```python
from build123d import *

# Parameters (mm, degrees)
F1_DEPTH = 100
F3_DEPTH = 100
F4_W     = 37.074
F4_H     = 23.256904
F4_H_2   = 25
F5_DEPTH = 150
F7_DEPTH = 25


with BuildPart() as f1:
    # F0 (on Front) → F1 (new body)
    with BuildSketch(Plane.XZ):
        Polygon((0, 90), (0, 0), (148.54021, 0), (148.54021, 110.875965), align=None)
    extrude(amount=F1_DEPTH)

    # F2 (on face) → F3 (cut)
    with BuildSketch(Plane.XZ.offset(100)):
        Polygon((7, 0), (40, 0), (148.54021, 0), (148.54021, 169.224784), (40, 169.224784), (40, 95.621633), (7, 57.987016), align=None)
    extrude(amount=-F3_DEPTH, mode=Mode.SUBTRACT)

    # F4 (on face) → F5 (cut)
    with BuildSketch(Plane(origin=(0, 0, 0), x_dir=(1, 0, 0), z_dir=(0, 0, -1))):
        with Locations((25.537, 8.371548)):
            Rectangle(F4_W, F4_H)
        with Locations((25.537, 42.5)):
            Rectangle(F4_W, F4_H_2)
        with Locations((25.537, 77.5)):
            Rectangle(F4_W, F4_H_2)
    extrude(amount=-F5_DEPTH, mode=Mode.SUBTRACT)

    # F6 (on face) → F7 (cut)
    with BuildSketch(Plane.YZ.offset(7)):
        with BuildLine():
            ThreePointArc((-8.5, 28.993508), (-25, 45.493508), (-41.5, 28.993508))
            Line((-41.5, 28.993508), (-8.5, 28.993508))
        make_face()
        with BuildLine():
            Line((-8.5, 28.993508), (-41.5, 28.993508))
            ThreePointArc((-41.5, 28.993508), (-25, 12.493508), (-8.5, 28.993508))
        make_face()
    extrude(amount=-F7_DEPTH, mode=Mode.SUBTRACT)


solid = f1.part
```
Can you work these out from the model? Positions are in its coordinate system, mm. A direction names the side the tool comes from. Round coordinates to 2 decimals unless told otherwise and drop trailing zeros. Loops run counter-clockwise (first coordinate to the right, second up) from the corner with the lowest first, then second, coordinate; pieces in that order, holes last. Notation, with made-up numbers: M -39,52 L -1,52 A15 ccw -1,66 Z; hole C 58.5,-6.5 d9. An arc over 180 degrees is marked long. Answer as a JSON object with one key per item and string values. Group by question number.
Q1. Imagine slicing it at C-C, the plane z = 43. Please give me the cut outline in (x, y), then the cut area to 3 significant figures.
Q2. Imagine slicing it at D-D, the plane y = -60. Please give me the cut outline in (x, z).
Q3. Please list where these lines run through material, in increasing order: L1, parallel to Y at x = 23.5, z = 77; L2, parallel to X at y = -30.5, z = 76; L3, parallel to Z at x = 4.5, y = -25.
Q4. Will these pins go through, and if not, where does the flat tip stop? pin 1 (5 mm diameter, centred on x = 11, z = 81, fed in from +Y); pin 2 (4 mm diameter, centred on y = -68.5, z = 44.5, fed in from +X).
Q5. Imagine slicing it at B-B, the plane x = 16. Please give me the cut outline in (y, z), then the cut area to 3 significant figures.
Q6. On a 3-axis mill with a long thin cutter (end or side, diameter ignored), from which of +Z, -Z, +X, -X, +Y, -Y can I reach the whole of each face in a straight line? I mean faces 5 (the flat face through (7, -49, 45)), 6 (the flat face through (20, -20, 81)), 7 (the flat face through (20, -65, 81)). Say none if no direction works.
Q7. Imagine slicing it at A-A, the plane y = -25. Please give me the cut outline in (x, z), then the cut area to 3 significant figures.
Q8. We'd pull the mould along Z, two halves only. Please class faces 1 (the flat face through (20, -30, 81)), 2 (the flat face through (15.836, -60.411, 92.226)), 3 (the flat face through (3, -49, 0)), 4 (the cylindrical face through (3.549, -40.242, 35.313)): +Z half, -Z half, draft (parallel to the pull), parting line (faces both ways), or undercut.
Findings:
{
 "1": {"outline": "M 0,-100 L 7,-100 L 7,-33.72 L 0,-33.72 Z; M 0,-16.28 L 7,-16.28 L 7,0 L 0,0 Z", "area": "578 mm2"},
 "2": {"outline": "M 0,0 L 7,0 L 7,57.99 L 40,95.62 L 0,90 Z"},
 "3": {"L1": "y = -100 to -90, -65 to -55, -30 to -20", "L2": "x = 0 to 7", "L3": "z = 0 to 12.49, 45.49 to 90.63"},
 "4": {"pin 1": "stops at y = -20", "pin 2": "stops at x = 7"},
 "5": {"outline": "M -100,68.25 L -90,68.25 L -90,92.25 L -100,92.25 Z; M -65,68.25 L -55,68.25 L -55,92.25 L -65,92.25 Z; M -30,68.25 L -20,68.25 L -20,92.25 L -30,92.25 Z", "area": "720 mm2"},
 "6": {"face 5": "-Z, +X", "face 6": "+Z, -Z, +X, +Y", "face 7": "+Z, -Z, +X"},
 "7": {"outline": "M 0,0 L 7,0 L 7,12.49 L 0,12.49 Z; M 0,45.49 L 7,45.49 L 7,57.99 L 40,95.62 L 0,90 Z", "area": "947 mm2"},
 "8": {"face 1": "draft", "face 2": "+Z half", "face 3": "-Z half", "face 4": "undercut"}
}
